from build123d import *

# Parameters (mm, degrees)
ESQUISSE1_W        = 25
ESQUISSE1_H        = 25
ESQUISSE1_R        = 1.25
BOSS_EXTRU_1_DEPTH = 8
CONG_1_R           = 2


with BuildPart() as part:
    # Esquisse1 → Boss.-Extru.1 (new body)
    with BuildSketch(Plane.XY):
        Rectangle(ESQUISSE1_W, ESQUISSE1_H)
        with Locations((-10, 10)):
            Circle(ESQUISSE1_R, mode=Mode.SUBTRACT)
        with Locations(Location((10, 10, 0), (0, 0, 180))):
            Circle(ESQUISSE1_R, mode=Mode.SUBTRACT)
        with Locations((10, -10)):
            Circle(ESQUISSE1_R, mode=Mode.SUBTRACT)
        with Locations(Location((-10, -10, 0), (0, 0, 180))):
            Circle(ESQUISSE1_R, mode=Mode.SUBTRACT)
    extrude(amount=BOSS_EXTRU_1_DEPTH)

    # Esquisse2 → Enlèvement de matière-Révolution1 (revolve, cut)
    with BuildSketch(Plane(origin=(0, 0, 0), x_dir=(0, 0, -1), z_dir=(1, 0, 0))):
        Polygon((-8, 0), (0, 0), (0, 10), (-1, 10), (-1, 11), (-8, 11), align=None)
    revolve(axis=Axis((0, 0, 8), (0, 0, 1)), mode=Mode.SUBTRACT)

    # Congé1
    cong_1_edges = [part.edges().sort_by_distance(p)[0] for p in [
        (-12.5, 12.5, 4),
        (12.5, 12.5, 4),
        (12.5, -12.5, 4),
        (-12.5, -12.5, 4),
    ]]
    fillet(cong_1_edges, radius=CONG_1_R)


solid = part.part
Work out the finished part from the listing and answer in its coordinate system (mm). A direction names the side the tool comes from. Round coordinates to 2 decimals unless told otherwise and drop trailing zeros. Write each loop counter-clockwise with the first axis right and the second up, starting at its lowest first coordinate (ties: lowest second). Pieces come first, ordered by that corner, then holes. Notation, with made-up numbers: (-11.75, 14) - (11.25, 14) arc R21 cw to (11.25, 28) - close; hole circle Ø6 at (50, 69.5). An arc over 180 degrees is marked (long way). Answer in a Markdown table with one row per item. Add a question column.
1. Given pin 1 (1.5 mm diameter, centred on x = 5, y = -8, fed in from +Z); pin 2 (4 mm diameter, centred on x = -10, y = -10, fed in from -Z), each flat-ended and moving along its own axis, determine where each tip first touches the part or whether it passes through.
2. For faces 1 (the cylindrical face through (10.74, -2.38, 4.55)), 2 (the cylindrical face through (11.25, 9.95, 3.94)), determine the directions among +Z, -Z, +X, -X, +Y, -Y from which every point of the face is accessible in a straight line to the end or side of a thin tool.
3. A cutting plane is placed at C-C, the plane y = 1.5. Determine the outline of the cut face in (x, z), and give its area (3 significant figures).
4. The mould has two halves that part along Y. Classify faces 3 (the flat face through (0, -12.5, 4)), 4 (the flat face through (10, -2, 1)), 5 (the flat face through (-12.5, 0, 4)), 6 (the cylindrical face through (-11.93, 11.9, 4.06)): +Y half, -Y half, draft (parallel to the pull), parting line (faces both ways), or undercut.
5. A cutting plane is placed at B-B, the plane x = -3. Determine the outline of the cut face in (y, z), and give its area (3 significant figures).
6. A cutting plane is placed at A-A, the plane z = 5.5. Determine the outline of the cut face in (x, y).
7. Find the intervals of material crossed by line 1 along Y through (x, z) = (10, 3.25); line 2 along X through (y, z) = (-9.75, 1.5); line 3 along Y through (x, z) = (9.25, 2.25), in increasing order. Write a range as from..to.
Worked out:
| question | item | result |
|---|---|---|
| 1 | pin 1 | z = 1 |
| 1 | pin 2 | z = 0 |
| 2 | face 1 | +Z |
| 2 | face 2 | +Z, -Z |
| 3 | outline | (-12.5, 0) - (-9.89, 0) - (-9.89, 1) - (-10.9, 1) - (-10.9, 8) - (-12.5, 8) - close; (9.89, 0) - (12.5, 0) - (12.5, 8) - (10.9, 8) - (10.9, 1) - (9.89, 1) - close |
| 3 | area | 27.7 mm^2 |
| 4 | face 3 | -Y half |
| 4 | face 4 | undercut |
| 4 | face 5 | draft |
| 4 | face 6 | +Y half |
| 5 | outline | (-12.5, 0) - (-9.54, 0) - (-9.54, 1) - (-10.58, 1) - (-10.58, 8) - (-12.5, 8) - close; (9.54, 0) - (12.5, 0) - (12.5, 8) - (10.58, 8) - (10.58, 1) - (9.54, 1) - close |
| 5 | area | 32.8 mm^2 |
| 6 | outline | (-12.5, -10.5) arc R2 ccw to (-10.5, -12.5) - (10.5, -12.5) arc R2 ccw to (12.5, -10.5) - (12.5, 10.5) arc R2 ccw to (10.5, 12.5) - (-10.5, 12.5) arc R2 ccw to (-12.5, 10.5) - close; hole circle Ø2.5 at (-10, -10); hole circle Ø2.5 at (-10, 10); hole circle Ø22 at (0, 0); hole circle Ø2.5 at (10, -10); hole circle Ø2.5 at (10, 10) |
| 7 | line 1 | -12.5..-11.25, -8.75..-4.58, 4.58..8.75, 11.25..12.5 |
| 7 | line 2 | -12.5..-11.22, -8.78..-5.09, 5.09..8.78, 11.22..12.5 |
| 7 | line 3 | -12.5..-11, -9..-5.95, 5.95..9, 11..12.5 |
